from build123d import *

# Parameters (mm, degrees)
F0_W     = 215.9
F0_H     = 50.8
F0_R     = 2.5527
F1_DEPTH = 25.4
F2_W     = 22.225
F2_H     = 47.625
F3_DEPTH = 215.901
F4_R     = 2.5527
F5_DEPTH = 50.801


with BuildPart() as f1:
    # F0 (on Front) → F1 (new body)
    with BuildSketch(Plane.XZ):
        Rectangle(F0_W, F0_H)
        with Locations((-82.55, -12.7)):
            Circle(F0_R, mode=Mode.SUBTRACT)
        with Locations((-57.15, -12.7)):
            Circle(F0_R, mode=Mode.SUBTRACT)
        with Locations((-31.75, -12.7)):
            Circle(F0_R, mode=Mode.SUBTRACT)
        with Locations((-6.35, -12.7)):
            Circle(F0_R, mode=Mode.SUBTRACT)
        with Locations((19.05, -12.7)):
            Circle(F0_R, mode=Mode.SUBTRACT)
        with Locations((44.45, -12.7)):
            Circle(F0_R, mode=Mode.SUBTRACT)
        with Locations((69.85, -12.7)):
            Circle(F0_R, mode=Mode.SUBTRACT)
        with Locations((95.25, -12.7)):
            Circle(F0_R, mode=Mode.SUBTRACT)
        with Locations((-82.55, 12.7)):
            Circle(F0_R, mode=Mode.SUBTRACT)
        with Locations((-57.15, 12.7)):
            Circle(F0_R, mode=Mode.SUBTRACT)
        with Locations((-31.75, 12.7)):
            Circle(F0_R, mode=Mode.SUBTRACT)
        with Locations((-6.35, 12.7)):
            Circle(F0_R, mode=Mode.SUBTRACT)
        with Locations((19.05, 12.7)):
            Circle(F0_R, mode=Mode.SUBTRACT)
        with Locations((44.45, 12.7)):
            Circle(F0_R, mode=Mode.SUBTRACT)
        with Locations((69.85, 12.7)):
            Circle(F0_R, mode=Mode.SUBTRACT)
        with Locations((95.25, 12.7)):
            Circle(F0_R, mode=Mode.SUBTRACT)
    extrude(amount=F1_DEPTH)

    # F2 (on face) → F3 (cut, through all)
    with BuildSketch(Plane(origin=(-107.95, 0, 0), x_dir=(0, -1, 0), z_dir=(-1, 0, 0))):
        with Locations((12.7, 0)):
            Rectangle(F2_W, F2_H)
    extrude(amount=-F3_DEPTH, mode=Mode.SUBTRACT)

    # F4 (on face) → F5 (cut, through all)
    with BuildSketch(Plane.XY.offset(25.4)):
        with Locations((-95.25, -12.7)):
            Circle(F4_R)
        with Locations((-57.15, -12.7)):
            Circle(F4_R)
        with Locations((-19.05, -12.7)):
            Circle(F4_R)
        with Locations((19.05, -12.7)):
            Circle(F4_R)
        with Locations((57.15, -12.7)):
            Circle(F4_R)
        with Locations((95.25, -12.7)):
            Circle(F4_R)
    extrude(amount=-F5_DEPTH, mode=Mode.SUBTRACT)


solid = f1.part
Read the model definition and answer for the solid it produces. Units are mm, in the model's axes. A direction names the side the tool comes from. Round coordinates to 2 decimals unless told otherwise and drop trailing zeros. Write each loop counter-clockwise with the first axis right and the second up, starting at its lowest first coordinate (ties: lowest second). Pieces come first, ordered by that corner, then holes. Notation, with made-up numbers: M -31,0 L 1,0 A24 ccw 1,17 Z; hole C -38,3 d2. An arc over 180 degrees is marked long. Use a Markdown table: item, result.
1) For a pull along Y with two mould halves and no side action, classify faces 3 (the cylindrical face through (42.42, -24.6, 11.15)), 4 (the cylindrical face through (-54.715, -11.933, 24.617)) as pulls with the +Y half, pulls with the -Y half, needs draft (parallel to the pull), parting line crosses it, or undercut.
Answers follow:
| item | result |
|---|---|
| face 3 | needs draft |
| face 4 | undercut |
2) The part is cut by section A-A (y = -7.5). Write down the section's boundary in (x, z).
Answers follow:
| item | result |
|---|---|
| outline | M -107.95,-25.4 L 107.95,-25.4 L 107.95,-23.81 L -107.95,-23.81 Z; M -107.95,23.81 L 107.95,23.81 L 107.95,25.4 L -107.95,25.4 Z |
3) The part is cut by section D-D (z = -18.5). Write down the section's boundary in (x, y).
Answers follow:
| item | result |
|---|---|
| outline | M -107.95,-25.4 L 107.95,-25.4 L 107.95,-23.81 L -107.95,-23.81 Z; M -107.95,-1.59 L 107.95,-1.59 L 107.95,0 L -107.95,0 Z |
4) The part is cut by section C-C (x = 52.5). Write down the section's boundary in (y, z).
Answers follow:
| item | result |
|---|---|
| outline | M -25.4,-25.4 L 0,-25.4 L 0,25.4 L -25.4,25.4 Z; hole M -23.81,-23.81 L -1.59,-23.81 L -1.59,23.81 L -23.81,23.81 Z |
5) The part is cut by section B-B (x = -95.25). Write down the section's boundary in (y, z), plus the area to 3 significant figures.
Answers follow:
| item | result |
|---|---|
| outline | M -25.4,-25.4 L -15.25,-25.4 L -15.25,-23.81 L -23.81,-23.81 L -23.81,23.81 L -15.25,23.81 L -15.25,25.4 L -25.4,25.4 Z; M -10.15,-25.4 L 0,-25.4 L 0,25.4 L -10.15,25.4 L -10.15,23.81 L -1.59,23.81 L -1.59,-23.81 L -10.15,-23.81 Z |
| area | 216 mm2 |
6) A tool of negligible diameter and unlimited length cuts with its end or side. For faces 1 (the flat face through (-2, -1.587, 0)), 2 (the cylindrical face through (54.6, -12.6, -24.6)), from which of +Z, -Z, +X, -X, +Y, -Y can it reach the whole face along a straight path? Write none if from no direction.
Answers follow:
| item | result |
|---|---|
| face 1 | +X, -X |
| face 2 | +Z, -Z |
7) Straight lines are drawn through the part: line 1 along Z through (x, y) = (19.05, -0.9); line 2 along Z through (x, y) = (21, -6.5); line 3 along Y through (x, z) = (-39, 14). For each, find the intervals that lie inside material, in ascending order. Write a range as [from, to].
Answers follow:
| item | result |
|---|---|
| line 1 | z = [-25.4, -15.25], [-10.15, 10.15], [15.25, 25.4] |
| line 2 | z = [-25.4, -23.81], [23.81, 25.4] |
| line 3 | y = [-25.4, -23.81], [-1.59, 0] |
